The listing builds one solid part. Answer for the finished solid, in the listing's coordinates (mm). A direction names the side the tool comes from. Round coordinates to 2 decimals unless told otherwise and drop trailing zeros. Order: outer loops, then holes, each group sorted by start corner. A loop starts at its lowest first (then second) coordinate and runs counter-clockwise, first axis right, second up. Notation, with made-up numbers: M 50.25,40 L 88.25,40 A8 cw 88.25,49 Z; hole C 5.5,52 d11. An arc over 180 degrees is marked long. Put each result on its own line as item: value. Start each with the question number.
1. Consider line 1 (X direction, y = 5, z = 0); line 2 (Y direction, x = 11, z = 0); line 3 (Y direction, x = -2.5, z = 0). Determine where each line is inside the solid, lowest interval first.
2. The part is cut by section D-D (x = 4). Give the vertices of the cut face in (y, z).
3. The part is cut by section C-C (y = 39). Give the vertices of the cut face in (x, z).
4. The part is cut by section B-B (z = 0). Count the separate pieces of the cut face and the enclosed holes in it, then the cut area to 3 significant figures.
5. The part is cut by section A-A (x = 19). Give the vertices of the cut face in (y, z).
6. Which of the six approach directions +Z, -Z, +X, -X, +Y, -Y give full straight-line access (tool end or side, diameter ignored) to faces 4 (the face through (16, 8, 0)), 5 (the face through (-8.5, 37, 2)), 6 (the face through (0.75, 42, 0))?
7. Each of these flat-tipped pins is pushed along its axis until it touches: pin 1 Ø6 at (y, z) = (31, 5) entering from +X; pin 2 Ø7 at (y, z) = (38.5, -2) entering from -X; pin 3 Ø8 at (x, z) = (19, 0) entering from +Y; pin 4 Ø3 at (x, z) = (-19, 0) entering from -Y. Where does it stop, or does it pass through?
8. The mould has two halves that part along Z. Classify faces 1 (the face through (0, 19, 0)), 2 (the face through (0, 17, -8)), 3 (the face through (-10.53, 42.47, -0.46)): +Z half, -Z half, draft (parallel to the pull), parting line (faces both ways), or undercut.
from build123d import *

# Parameters (mm, degrees)
SALIENTE_EXTRUIR1_DEPTH = 8
CROQUIS3_R              = 2.5
CORTAR_EXTRUIR1_DEPTH   = 9
REDONDEO1_R             = 1
CROQUIS4_R              = 2
CORTAR_EXTRUIR2_DEPTH   = 37.5
CROQUIS5_R              = 3.5
CORTAR_EXTRUIR3_DEPTH   = 4


with BuildPart() as part:
    # Croquis1 → Saliente-Extruir1 (new body, symmetric)
    with BuildSketch(Plane.XY):
        with BuildLine():
            Line((-24, 0), (24, 0))
            Line((24, 0), (24, 8))
            Line((24, 8), (12.5, 8))
            Line((12.5, 8), (12.5, 44))
            Line((12.5, 44), (0.75, 44))
            Line((0.75, 44), (0.75, 34.964766161))
            ThreePointArc((0.75, 34.964766161), (0, 19), (-0.75, 34.964766161))
            Line((-0.75, 34.964766161), (-0.75, 44))
            Line((-0.75, 44), (-12.5, 44))
            Line((-12.5, 44), (-12.5, 8))
            Line((-12.5, 8), (-24, 8))
            Line((-24, 8), (-24, 0))
        make_face()
    extrude(amount=SALIENTE_EXTRUIR1_DEPTH, both=True)

    # Croquis3 → Cortar-Extruir1 (cut, through all)
    with BuildSketch(Plane(origin=(0, 8, 0), x_dir=(1, 0, 0), z_dir=(0, 1, 0))):
        with Locations((-19, 0)):
            Circle(CROQUIS3_R)
        with Locations((19, 0)):
            Circle(CROQUIS3_R)
    extrude(amount=-CORTAR_EXTRUIR1_DEPTH, mode=Mode.SUBTRACT)

    # Redondeo1
    redondeo1_edges = [part.edges().sort_by_distance(p)[0] for p in [
        (-12.5, 8, 0),
        (12.5, 8, 0),
    ]]
    fillet(redondeo1_edges, radius=REDONDEO1_R)

    # Croquis4 → Cortar-Extruir2 (cut, through all)
    with BuildSketch(Plane.ZY.offset(12.5)):
        with Locations((0, 39)):
            Circle(CROQUIS4_R)
    extrude(amount=-CORTAR_EXTRUIR2_DEPTH, mode=Mode.SUBTRACT)

    # Croquis5 → Cortar-Extruir3 (cut)
    with BuildSketch(Plane.ZY.offset(12.5)):
        with Locations((0, 39)):
            Circle(CROQUIS5_R)
    extrude(amount=-CORTAR_EXTRUIR3_DEPTH, mode=Mode.SUBTRACT)


solid = part.part
Resolved:
1. line 1: -24 to -21.5, -16.5 to 16.5, 21.5 to 24
1. line 2: 0 to 37, 41 to 44
1. line 3: 0 to 19.4, 34.6 to 37, 41 to 44
2. outline: M 0,-8 L 20.07,-8 L 20.07,8 L 0,8 Z; M 33.93,-8 L 44,-8 L 44,8 L 33.93,8 Z; hole C 39,0 d4
3. outline: M -12.5,-8 L -0.75,-8 L -0.75,-2 L -8.5,-2 L -8.5,-3.5 L -12.5,-3.5 Z; M -12.5,3.5 L -8.5,3.5 L -8.5,2 L -0.75,2 L -0.75,8 L -12.5,8 Z; M 0.75,-8 L 12.5,-8 L 12.5,-2 L 0.75,-2 Z; M 0.75,2 L 12.5,2 L 12.5,8 L 0.75,8 Z
4. separate pieces: 5
4. enclosed holes: 0
4. area: 884 mm2
5. outline: M 0,-8 L 8,-8 L 8,-2.5 L 0,-2.5 Z; M 0,2.5 L 8,2.5 L 8,8 L 0,8 Z
6. face 4: +Z, -Z, +X, +Y
6. face 5: -X
6. face 6: +Z, -Z, +Y
7. pin 1: x = 12.5
7. pin 2: x = -12.5
7. pin 3: y = 8
7. pin 4: through
8. face 1: draft
8. face 2: -Z half
8. face 3: undercut
